Could you check a few things on this model? Use its own coordinates, in mm. A direction names the side the tool comes from. Round coordinates to 2 decimals unless told otherwise and drop trailing zeros. Loops run counter-clockwise (first coordinate to the right, second up) from the corner with the lowest first, then second, coordinate; pieces in that order, holes last. Notation, with made-up numbers: M 51,-13.75 L 104,-13.75 A18 ccw 104,21.25 Z; hole C 19,21.5 d9. An arc over 180 degrees is marked long. One line per item, written item: value. Start each with the question number.
Q1. Please list where these lines run through material, in increasing order: line 1 along X through (y, z) = (10, 8.75); line 2 along Y through (x, z) = (-14, 10.5); line 3 along X through (y, z) = (4, 15.75).
Q2. Which directions (+Z, -Z, +X, -X, +Y, -Y) give clear straight access to the entire face, cutting with the end or side of a thin tool? Please do faces 1 (the face through (-12.7, 13, 13)), 2 (the face through (-32, 6, 6)), 3 (the face through (-25, 19, 12.7)), 4 (the face through (-19, 12.7, 6)), 5 (the face through (-6, 19, 25.4)).
Q3. Imagine slicing it at B-B (z = 2.75). Please give me the cut outline in (x, y), then the cut area to 3 significant figures.
Q4. Imagine slicing it at D-D (y = 8). Please give me the cut outline in (x, z), then the cut area to 3 significant figures.
Q5. I'm going to push flat-ended pins straight in: pin 1 Ø6.5 at (x, y) = (-21.5, 19.5) entering from +Z; pin 2 Ø1.5 at (x, z) = (-18.5, 14) entering from +Y. Where does each tip first touch, or does it pass through?
Q6. Imagine slicing it at C-C (x = -3). Please give me the cut outline in (y, z), then the cut area to 3 significant figures.
Q7. Imagine slicing it at A-A (y = 12). Please give me the cut outline in (x, z).
from build123d import *

# Parameters (mm, degrees)
F1_DEPTH = 38.1
F2_W     = 25.4
F2_H     = 12.7
F3_DEPTH = 25.4
F4_W     = 12.7
F4_H     = 12.7
F5_DEPTH = 12.7
F7_DEPTH = 12.7


with BuildPart() as f1:
    # F0 (on Right) → F1 (new body)
    with BuildSketch(Plane.YZ):
        Polygon((0, 12.7), (0, 0), (25.4, 0), (25.4, 25.4), (12.7, 25.4), align=None)
    extrude(amount=-F1_DEPTH)

    # F2 (on face) → F3 (cut)
    with BuildSketch(Plane(origin=(0, 25.4, 0), x_dir=(-1, 0, 0), z_dir=(0, 1, 0))):
        with Locations((25.4, 19.05)):
            Rectangle(F2_W, F2_H)
    extrude(amount=-F3_DEPTH, mode=Mode.SUBTRACT)

    # F4 (on face) → F5 (cut)
    with BuildSketch(Plane.XZ):
        with Locations((-19.05, 6.35)):
            Rectangle(F4_W, F4_H)
    extrude(amount=-F5_DEPTH, mode=Mode.SUBTRACT)

    # F6 (on face) → F7 (cut)
    with BuildSketch(Plane(origin=(-38.1, 0, 0), x_dir=(0, -1, 0), z_dir=(-1, 0, 0))):
        Polygon((-12.7, 12.7), (0, 0), (0, 12.7), align=None)
    extrude(amount=-F7_DEPTH, mode=Mode.SUBTRACT)


solid = f1.part
Report:
1. line 1: x = -38.1 to -25.4, -12.7 to 0
1. line 2: y = 12.7 to 25.4
1. line 3: x = -12.7 to 0
2. face 1: +Z, -Y
2. face 2: +Z, -X, -Y
2. face 3: +Z, -X, +Y, -Y
2. face 4: +Z, -Z, -Y
2. face 5: +Z, +X, -X, +Y, -Y
3. outline: M -38.1,2.75 L -25.4,2.75 L -25.4,12.7 L -12.7,12.7 L -12.7,0 L 0,0 L 0,25.4 L -38.1,25.4 Z
3. area: 772 mm²
4. outline: M -38.1,0 L -25.4,0 L -25.4,8 L -38.1,8 Z; M -12.7,0 L 0,0 L 0,20.7 L -12.7,20.7 Z
4. area: 364 mm²
5. pin 1: stops at z = 12.7
5. pin 2: passes through
6. outline: M 0,0 L 25.4,0 L 25.4,25.4 L 12.7,25.4 L 0,12.7 Z
6. area: 565 mm²
7. outline: M -38.1,0 L -25.4,0 L -25.4,12 L -38.1,12 Z; M -12.7,0 L 0,0 L 0,24.7 L -12.7,24.7 Z
